The figure shows three views and two pictorial views of one solid part (mm, origin at its lowest corner). Answer the questions. A direction names the side the tool comes from. Round coordinates to 2 decimals unless told otherwise and drop trailing zeros. Order: outer loops, then holes, each group sorted by start corner. A loop starts at its lowest first (then second) coordinate and runs counter-clockwise, first axis right, second up. Notation, with made-up numbers: (62.25, 10) -> (77.25, 10) arc R14 ccw to (77.25, 34) -> close; hole circle Ø10 at (-21, 26). An arc over 180 degrees is marked (long way). Answer as a JSON object with one key per item and string values. Group by question number.
Item 1: Given P1, Ø2.5, axis at x = 2, y = 7, coming from the -Z side; P2, Ø2.5, axis at x = 2, z = 6.5, coming from the +Y side (1 decimal); P3, Ø1.5, axis at y = 5.5, z = 6.5, coming from the -X side, each flat-ended and moving along its own axis, determine where each tip first touches the part or whether it passes through.
Item 2: Section B-B, the plane y = 8.5 is taken. Write down the section's boundary in (x, z).
Item 3: The mould has two halves that part along X. Classify the marked faces 3, 4 and 5: pulls with the +X half, pulls with the -X half, needs draft (parallel to the pull), parting line crosses it, or undercut.
Item 4: Section A-A, the plane z = 3.25 is taken. Write down the section's boundary in (x, y) (1 decimal).
Item 5: Section D-D, the plane y = 2.5 is taken. Count the separate pieces of the cut face and the enclosed holes in it.
Item 6: Consider probe 1 along Y at (x, z) = (2.45, 16.5); probe 2 along X at (y, z) = (2.2, 3.25) (1 decimal); probe 3 along Z at (x, y) = (2.75, 1.5). Determine where each line is inside the solid, lowest interval first. Write a range as from..to.
Item 7: For the marked faces 1 and 2, determine the directions among +Z, -Z, +X, -X, +Y, -Y from which every point of the face is accessible in a straight line to the end or side of a thin tool.
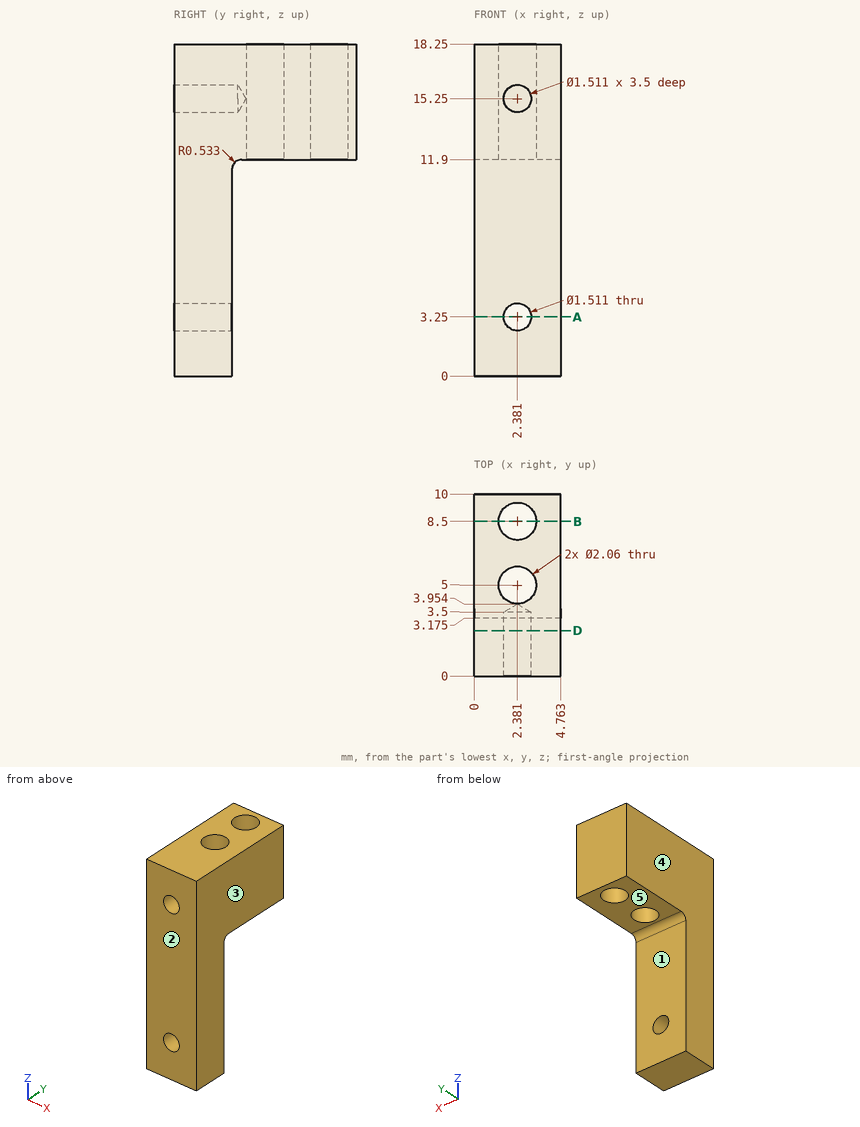
Values found:
{
 "1": {"P1": "z = 11.9", "P2": "y = 3.2", "P3": "through"},
 "2": {"outline": "(0, 11.9) -> (1.35, 11.9) -> (1.35, 18.25) -> (0, 18.25) -> close; (3.41, 11.9) -> (4.76, 11.9) -> (4.76, 18.25) -> (3.41, 18.25) -> close"},
 "3": {"face 3": "pulls with the +X half", "face 4": "pulls with the -X half", "face 5": "needs draft"},
 "4": {"outline": "(0, 0) -> (1.6, 0) -> (1.6, 3.2) -> (0, 3.2) -> close; (3.1, 0) -> (4.8, 0) -> (4.8, 3.2) -> (3.1, 3.2) -> close"},
 "5": {"separate pieces": "1", "enclosed holes": "2"},
 "6": {"probe 1": "0..3.97, 6.03..7.47, 9.53..10", "probe 2": "0..1.6, 3.1..4.8", "probe 3": "0..2.59, 3.91..14.59, 15.91..18.25"},
 "7": {"face 1": "-Z, +X, -X, +Y", "face 2": "+Z, -Z, +X, -X, -Y"}
}
